Can you work these out from the drawing? Everything is in mm from the part's minimum corner. Give positions to 0.01 mm unless a question says otherwise; leave off trailing zeros. Order: outer loops, then holes, each group sorted by start corner. A loop starts at its lowest first (then second) coordinate and runs counter-clockwise, first axis right, second up. Notation, with made-up numbers: (-6, 70) -> (5, 70) arc R25 ccw to (5, 108) -> close; hole circle Ø3 at (30, 51.5). An arc over 180 degrees is marked (long way). Answer as CSV lines item,"result". Start each with the question number.
(1) I want a section at A-A (z = 5.75). Please give me the cut outline in (x, y), plus the area to 3 significant figures.
(2) I need wall thicknesses on L1, parallel to Y at x = 2.25, z = 5.75; L2, parallel to X at y = 60, z = 5; L3, parallel to Y at x = 8.75, z = 4.5. Which ranges of each line are inside material? Lowest first, please.
(3) I want a section at C-C (x = 1). Please give me the cut outline in (y, z), plus the area to 3 significant figures.
(4) I want a section at D-D (y = 60). Please give me the cut outline in (x, z), plus the area to 3 significant figures.
(5) We'd pull the mould along Y, two halves only. Please class the marked faces 1, 2, 3 and 4: released by +Y, released by -Y, zero draft, split by the parting line, or undercut.
(6) I want a section at B-B (y = 92.5). Please give me the cut outline in (x, z), plus the area to 3 significant figures.
(7) Will this pin go through, and if not, where does the flat tip stop? pin 1 Ø3.5 at (y, z) = (92.5, 5.75) entering from +X.
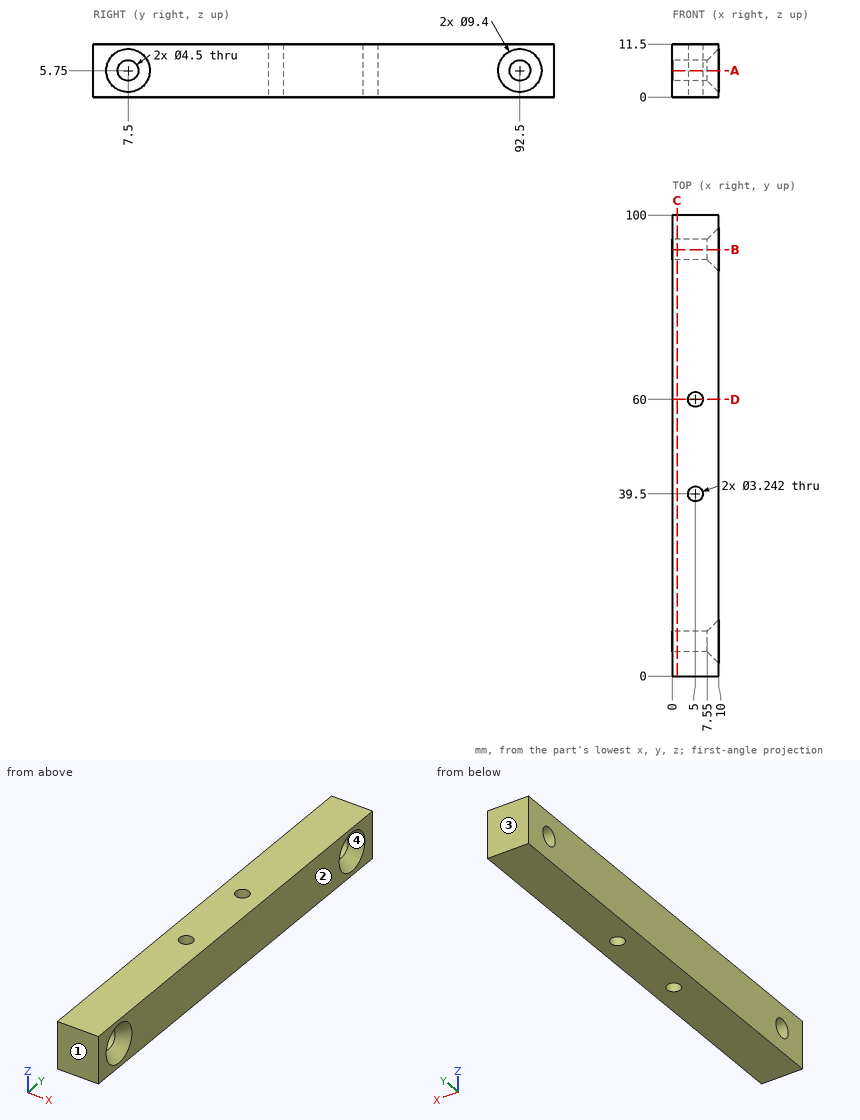
Final values:
1,outline,"(0, 0) -> (10, 0) -> (10, 2.8) -> (7.55, 5.25) -> (0, 5.25) -> close; (0, 9.75) -> (7.55, 9.75) -> (10, 12.2) -> (10, 87.8) -> (7.55, 90.25) -> (0, 90.25) -> close; (0, 94.75) -> (7.55, 94.75) -> (10, 97.2) -> (10, 100) -> (0, 100) -> close; hole circle Ø3.24 at (5, 39.5); hole circle Ø3.24 at (5, 60)"
1,area,"881 mm²"
2,L1,"0 to 5.25, 9.75 to 90.25, 94.75 to 100"
2,L2,"0 to 3.38, 6.62 to 10"
2,L3,"0 to 4.28, 10.72 to 89.28, 95.72 to 100"
3,outline,"(0, 0) -> (100, 0) -> (100, 11.5) -> (0, 11.5) -> close; hole circle Ø4.5 at (7.5, 5.75); hole circle Ø4.5 at (92.5, 5.75)"
3,area,"1,120 mm²"
4,outline,"(0, 0) -> (3.38, 0) -> (3.38, 11.5) -> (0, 11.5) -> close; (6.62, 0) -> (10, 0) -> (10, 11.5) -> (6.62, 11.5) -> close"
4,area,"77.7 mm²"
5,face 1,"released by -Y"
5,face 2,"zero draft"
5,face 3,"released by +Y"
5,face 4,"undercut"
6,outline,"(0, 0) -> (10, 0) -> (10, 1.05) -> (7.55, 3.5) -> (0, 3.5) -> close; (0, 8) -> (7.55, 8) -> (10, 10.45) -> (10, 11.5) -> (0, 11.5) -> close"
6,area,"64.0 mm²"
7,pin 1,"through"
